The listing builds one solid part. Answer for the finished solid, in the listing's coordinates (mm). Face numbers are marked on the shaded views. A direction names the side the tool comes from. Round coordinates to 2 decimals unless told otherwise and drop trailing zeros. Order: outer loops, then holes, each group sorted by start corner. A loop starts at its lowest first (then second) coordinate and runs counter-clockwise, first axis right, second up. Notation, with made-up numbers: M -37,80 L 8,80 A20 cw 8,99 Z; hole C -24.75,45 d7. An arc over 180 degrees is marked long. Write item = value, one per line. Start each with the question number.
(1) Which of the six approach directions +Z, -Z, +X, -X, +Y, -Y give full straight-line access (tool end or side, diameter ignored) to the marked faces 4 and 5?
(2) Straight lines are drawn through the part: probe 1 along Y at (x, z) = (0, 26.5); probe 2 along X at (y, z) = (-15, 24); probe 3 along Y at (x, z) = (4.5, 45). For each, find the intervals that lie inside material, in ascending order. Write a range as from..to.
(3) For a pull along X with two mould halves and no side action, classify the marked faces 1, 2 and 3 as released by +X, released by -X, zero draft, split by the parting line, or undercut.
(4) A cutting plane is placed at C-C, the plane z = 4.5. Determine the outline of the cut face in (x, y).
(5) A cutting plane is placed at A-A, the plane y = 0. Determine the outline of the cut face in (x, z).
(6) A cutting plane is placed at B-B, the plane x = 0. Determine the outline of the cut face in (y, z), and give its area (3 significant figures).
(7) Each of these flat-tipped pins is pushed along its axis until it touches: pin 1 (1.4 mm diameter, centred on x = 21.5, z = 33, fed in from -Y); pin 2 (2 mm diameter, centred on x = -10, z = 9.5, fed in from +Y); pin 3 (5 mm diameter, centred on x = 21, z = 25.5, fed in from +Y); pin 4 (5 mm diameter, centred on y = 1.5, z = 18, fed in from -X). Where does it stop, or does it pass through?
Autodesk Inventor part; units mm, degrees
ref_plane "YZ Plane" through (0, 0, 0) normal (1, 0, 0) x (0, 1, 0)
ref_plane "XZ Plane" through (0, 0, 0) normal (0, 1, 0) x (-1, 0, 0)
ref_plane "XY Plane" through (0, 0, 0) normal (0, 0, 1) x (1, 0, 0)
ref_plane "Płaszczyzna konstrukcyjna1" through (0, 0, 0) normal (0, 0, 1) x (1, 0, 0)
sketch "Szkic1" plane through (0, 0, 0) normal (0, 0, 1) x (1, 0, 0)
  arc A0 (19.3649, 5) -> (19.3649, -5) centre (0, 0) ccw
  line L0 (19.3649, 5) -> (24, 5)
  line L1 (24, 5) -> (24, -5)
  line L2 (24, -5) -> (19.3649, -5)
  circle A1 centre (0, 0) radius 30
  dimension "d0" = 60
extrude "Wyciągnięcie proste1" add sketch "Szkic1" along normal blind 48
chamfer "Faza1" distance 2 angle 45 1 edges at (-30, 0, 48)
chamfer "Faza2" distance 1 angle 45 1 edges at (-20, 0, 48)
properties material "Stal nierdzewna"
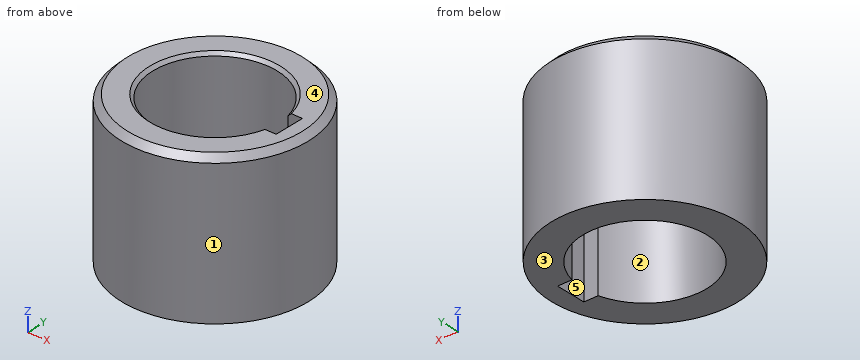
Reported:
q1.face_4 = +Z, +X, -X, +Y, -Y
q1.face_5 = +Z, -Z
q2.probe_1 = -30..-20, 20..30
q2.probe_2 = -25.98..-13.23, 13.23..25.98
q2.probe_3 = -29.66..-19.49, 19.49..29.66
q3.face_1 = split by the parting line
q3.face_2 = undercut
q3.face_3 = zero draft
q4.outline = C 0,0 d60; hole M 19.36,-5 L 24,-5 L 24,5 L 19.36,5 A20 ccw long Z
q5.outline = M -30,0 L -20,0 L -20,47 L -21,48 L -28,48 L -30,46 Z; M 24,0 L 30,0 L 30,46 L 28,48 L 24,48 Z
q6.outline = M -30,0 L -20,0 L -20,47 L -21,48 L -28,48 L -30,46 Z; M 20,0 L 30,0 L 30,46 L 28,48 L 21,48 L 20,47 Z
q6.area = 955 mm²
q7.pin_1 = -21.62
q7.pin_2 = 28.62
q7.pin_3 = 23.62
q7.pin_4 = -30
